from build123d import *

# Parameters (mm, degrees)
F1_DEPTH = 0.4
F3_DEPTH = 0.4
F5_DEPTH = 0.6
F6_R     = 0.5


with BuildPart() as f1:
    # F0 (on Top) → F1 (new body)
    with BuildSketch(Plane.XY):
        Polygon((0, 14), (0, 0), (5.78, 0), (11.56, 0), (11.56, 14), (10.93, 14.75), (10.93, 16.25), (11.56, 17), (11.56, 19.5), (5.78, 19.5), (0, 19.5), (0, 17), (0.63, 16.25), (0.63, 14.75), align=None)
        Polygon((10.53, 6.5), (9.53, 5.5), (1.03, 5.5), (1.03, 18.5), (10.53, 18.5), align=None, mode=Mode.SUBTRACT)
    extrude(amount=F1_DEPTH)

    # F2 (on face) → F3 (join)
    with BuildSketch(Plane(origin=(0, 0, 0), x_dir=(1, 0, 0), z_dir=(0, 0, -1))):
        Polygon((0.63, -2.3095843679), (0.63, -19.5), (1.68, -19.5), (1.68, -3), (5.78, -3), (9.88, -3), (9.88, -19.5), (10.93, -19.5), (10.93, -2.3095843679), (10.53, -1.5567192639), (10.53, 0), (5.78, 0), (1.03, 0), (1.03, -1.5567192639), align=None)
    extrude(amount=F3_DEPTH)

    # F4 (on face) → F5 (join)
    with BuildSketch(Plane.XZ):
        with BuildLine():
            Line((-2.2, 0.4), (-2.85, 0.4))
            Line((-2.85, 0.4), (-2.85, -0.4))
            Line((-2.85, -0.4), (12.86, -0.4))
            Line((12.86, -0.4), (12.86, 0.4))
            Line((12.86, 0.4), (-1.2, 0.4))
            ThreePointArc((-1.2, 0.4), (-1.7, -0.1), (-2.2, 0.4))
        make_face()
    extrude(amount=F5_DEPTH)

    # F6
    f6_edges = [f1.edges().sort_by_distance(p)[0] for p in [
        (11.56, 19.5, 0.2),
        (11.56, 17, 0.2),
        (10.93, 16.25, 0.2),
        (10.93, 14.75, 0.2),
        (11.56, 14, 0.2),
        (0, 19.5, 0.2),
        (0, 17, 0.2),
        (0.63, 16.25, 0.2),
        (0, 14, 0.2),
        (0.63, 14.75, 0.2),
        (9.88, 3, -0.2),
        (1.68, 3, -0.2),
        (10.93, 19.5, -0.2),
        (9.88, 19.5, -0.2),
        (1.68, 19.5, -0.2),
        (0.63, 19.5, -0.2),
        (10.53, 0, -0.2),
        (1.03, 0, -0.2),
    ]]
    fillet(f6_edges, radius=F6_R)


solid = f1.part
Read the model definition and answer for the solid it produces. Units are mm, in the model's axes. A direction names the side the tool comes from. Round coordinates to 2 decimals unless told otherwise and drop trailing zeros. Loops run counter-clockwise (first coordinate to the right, second up) from the corner with the lowest first, then second, coordinate; pieces in that order, holes last.
Q1. Determine the mould class of faces 5 (the face through (10.04, 6.01, 0.2)), 6 (the face through (6, 4, 0)) for opening direction Y: released by +Y, released by -Y, zero draft, split by the parting line, or undercut.
Q2. Consider probe 1 along X at (y, z) = (15, 0.35); probe 2 along X at (y, z) = (8, 0.2); probe 3 along Y at (x, z) = (-1, 0.2). Determine where each line is inside the solid, lowest interval first.
Q3. Which of the six approach directions +Z, -Z, +X, -X, +Y, -Y give full straight-line access (tool end or side, diameter ignored) to faces 1 (the face through (11.2, 18.2, 0)), 2 (the face through (6, 5, 0.4)), 3 (the face through (0.3, 18.2, 0)), 4 (the face through (6, 19, 0))?
Q4. Section C-C on x = -1.7 is taken. Write down the section's boundary in (y, z), and give its area (3 significant figures).
Q5. Each of these flat-tipped pins is pushed along its axis until it touches: pin 1 (1.1 mm diameter, centred on x = 3.5, y = 19, fed in from -Z); pin 2 (0.7 mm diameter, centred on x = 10, y = 12.5, fed in from +Z). Where does it stop, or does it pass through?
Q6. Section B-B on y = 9 is taken. Write down the section's boundary in (x, z), and give its area (3 significant figures).
Q7. Section A-A on z = -0.25 is taken. Write down the section's boundary in (x, y), and give its area (3 significant figures).
Output:
1. face 5: undercut
1. face 6: zero draft
2. probe 1: x = 0.63 to 1.03, 10.53 to 10.93
2. probe 2: x = 0 to 1.03, 10.53 to 11.56
2. probe 3: y = -0.6 to 0
3. face 1: -Z, +X, +Y
3. face 2: +Z, +X, -X, +Y, -Y
3. face 3: -Z, -X, +Y
3. face 4: -Z, +Y
4. outline: (-0.6, -0.4) - (0, -0.4) - (0, -0.1) - (-0.6, -0.1) - close
4. area: 0.180 mm2
5. pin 1: stops at z = 0
5. pin 2: stops at z = 0
6. outline: (0, 0) - (0.63, 0) - (0.63, -0.4) - (1.68, -0.4) - (1.68, 0) - (1.03, 0) - (1.03, 0.4) - (0, 0.4) - close; (9.88, -0.4) - (10.93, -0.4) - (10.93, 0) - (11.56, 0) - (11.56, 0.4) - (10.53, 0.4) - (10.53, 0) - (9.88, 0) - close
6. area: 1.66 mm2
7. outline: (-2.85, -0.6) - (12.86, -0.6) - (12.86, 0) - (11.03, 0) arc R0.5 cw to (10.53, 0.5) - (10.53, 1.56) - (10.93, 2.31) - (10.93, 19) arc R0.5 ccw to (10.43, 19.5) - (10.38, 19.5) arc R0.5 ccw to (9.88, 19) - (9.88, 3.5) arc R0.5 cw to (9.38, 3) - (2.18, 3) arc R0.5 cw to (1.68, 3.5) - (1.68, 19) arc R0.5 ccw to (1.18, 19.5) - (1.13, 19.5) arc R0.5 ccw to (0.63, 19) - (0.63, 2.31) - (1.03, 1.56) - (1.03, 0.5) arc R0.5 cw to (0.53, 0) - (-2.85, 0) - close
7. area: 73.4 mm2
